```python
from build123d import *

# Parameters (mm, degrees)
F0_W     = 38.1
F0_H     = 50.8
F1_DEPTH = 6.35
F2_R     = 3.175
F3_DEPTH = 6.351
F4_W     = 3.175
F4_H     = 12.7
F5_DEPTH = 6.351
F6_W     = 6.35
F6_H     = 12.7
F7_DEPTH = 6.351


with BuildPart() as f1:
    # F0 (on Front) → F1 (new body)
    with BuildSketch(Plane.XZ):
        with Locations((-1.309197, 31.935506)):
            Rectangle(F0_W, F0_H)
    extrude(amount=F1_DEPTH)

    # F2 (on face) → F3 (cut, through all)
    with BuildSketch(Plane(origin=(0, 0, 0), x_dir=(-1, 0, 0), z_dir=(0, 1, 0))):
        with Locations((1.309197, 48.445506)):
            Circle(F2_R)
    extrude(amount=-F3_DEPTH, mode=Mode.SUBTRACT)

    # F4 (on face) → F5 (cut, through all)
    with BuildSketch(Plane.XZ.offset(6.35)):
        with Locations((-18.771697, 12.885506)):
            Rectangle(F4_W, F4_H)
        with Locations((16.153303, 12.885506)):
            Rectangle(F4_W, F4_H)
    extrude(amount=-F5_DEPTH, mode=Mode.SUBTRACT)

    # F6 (on face) → F7 (cut, through all)
    with BuildSketch(Plane.XZ.offset(6.35)):
        with Locations((-1.309197, 12.885506)):
            Rectangle(F6_W, F6_H)
    extrude(amount=-F7_DEPTH, mode=Mode.SUBTRACT)


solid = f1.part
```
For this review, take the finished solid that the model builds, in its own axes (mm). A direction names the side the tool comes from. Round coordinates to 2 decimals unless told otherwise and drop trailing zeros. Write each loop counter-clockwise with the first axis right and the second up, starting at its lowest first coordinate (ties: lowest second). Pieces come first, ordered by that corner, then holes. Notation, with made-up numbers: (71, -34.75) -> (91, -34.75) arc R28 cw to (91, -10.75) -> close; hole circle Ø8 at (68, -4). An arc over 180 degrees is marked (long way). Use one line per item in the form item = value.
1) Mouldability with a two-part tool opening along X and no side actions: class faces 1 (the flat face through (17.741, -3, 38)), 2 (the cylindrical face through (-0.621, -3.131, 45.346)), 3 (the flat face through (16, -3, 19.236)) as +X half, -X half, draft (parallel to the pull), parting line (faces both ways), or undercut.
Found:
face_1 = +X half
face_2 = undercut
face_3 = draft
2) Take a section at A-A, the plane z = 15. Write out the cut boundary in (x, y).
Found:
outline = (-17.18, -6.35) -> (-4.48, -6.35) -> (-4.48, 0) -> (-17.18, 0) -> close; (1.87, -6.35) -> (14.57, -6.35) -> (14.57, 0) -> (1.87, 0) -> close
3) Take a section at D-D, the plane x = 15.5. Write out the cut boundary in (y, z).
Found:
outline = (-6.35, 19.24) -> (0, 19.24) -> (0, 57.34) -> (-6.35, 57.34) -> close
4) Tool access review of faces 4 (the flat face through (-19, -3, 19.236)), 5 (the flat face through (1.866, -3, 13)), 6 (the flat face through (14.566, -3, 13)): name each direction out of +Z, -Z, +X, -X, +Y, -Y from which nothing blocks a thin tool from reaching the whole face with its end or side.
Found:
face_4 = -Z, -X, +Y, -Y
face_5 = -Z, +Y, -Y
face_6 = -Z, +X, +Y, -Y
5) Take a section at B-B, the plane x = -0.5. Write out the cut boundary in (y, z), and give its area (3 significant figures).
Found:
outline = (-6.35, 19.24) -> (0, 19.24) -> (0, 45.38) -> (-6.35, 45.38) -> close; (-6.35, 51.52) -> (0, 51.52) -> (0, 57.34) -> (-6.35, 57.34) -> close
area = 203 mm2
6) Clearance check with flat-ended pins moving along their axes: pin 1 (1.9 mm diameter, centred on x = -1, y = -2.5, fed in from -Z); pin 2 (2 mm diameter, centred on x = 5.5, z = 13, fed in from +Y); pin 3 (5.5 mm diameter, centred on x = -1.31, z = 48.45, fed in from -Y); pin 4 (3 mm diameter, centred on y = -4, z = 10, fed in from +X). State where each tip first meets the part, or that it passes through.
Found:
pin_1 = 19.24
pin_2 = 0
pin_3 = through
pin_4 = 14.57
7) To check wall thickness, follow L1, parallel to Z at x = 0.5, y = -0.5; L2, parallel to Z at x = -2, y = -0.75; L3, parallel to X at y = -3.25, z = 50.5. State the ranges of each line that lie inside material, in increasing order. Write a range as from..to.
Found:
L1 = 19.24..45.84, 51.05..57.34
L2 = 19.24..45.35, 51.54..57.34
L3 = -20.36..-3.73, 1.11..17.74
